```python
from build123d import *

# Parameters (mm, degrees)
F1_DEPTH = 15
F2_R     = 1
F3_R     = 1


with BuildPart() as f1:
    # F0 (on Front) → F1 (new body)
    with BuildSketch(Plane.XZ):
        Polygon((-4.5, 0), (-4.5, -18.7), (-2.75, -17.2), (-3.25, -7.2), (3.25, -7.2), (2.75, -17.2), (4.5, -18.7), (4.5, -1), (4.5, 0), align=None)
    extrude(amount=F1_DEPTH)

    # F2
    f2_edges = [f1.edges().sort_by_distance(p)[0] for p in [
        (-2.75, -7.5, -17.2),
        (-4.5, -7.5, 0),
        (4.5, -7.5, 0),
        (2.75, -7.5, -17.2),
    ]]
    fillet(f2_edges, radius=F2_R)

    # F3
    f3_edges = [f1.edges().sort_by_distance(p)[0] for p in [
        (-3.25, -7.5, -7.2),
        (3.25, -7.5, -7.2),
    ]]
    fillet(f3_edges, radius=F3_R)


solid = f1.part
```
Geometry check sheet. Reference: the model listing, model coordinates, mm. A direction names the side the tool comes from. Give positions to 0.01 mm unless a question says otherwise; leave off trailing zeros. Write each loop counter-clockwise with the first axis right and the second up, starting at its lowest first coordinate (ties: lowest second). Pieces come first, ordered by that corner, then holes. Notation, with made-up numbers: (56.5, 27) - (70.5, 27) arc R21 cw to (70.5, 57) - close; hole circle Ø5 at (-30, 12). An arc over 180 degrees is marked (long way). Use a Markdown table: item, result.
Q1. Thickness scan on L1, parallel to Z at x = 0, y = -11.5; L2, parallel to X at y = -10.5, z = -11; L3, parallel to X at y = -0.5, z = -16.25. Record the ranges inside material, lowest first. Write a range as [from, to].
Computed:
| item | result |
|---|---|
| L1 | z = [-7.2, 0] |
| L2 | x = [-4.5, -3.06], [3.06, 4.5] |
| L3 | x = [-4.5, -2.8], [2.8, 4.5] |
Q2. Go/stop test with flat-tipped pins: P1, Ø1, axis at x = 2.5, z = -6.5, coming from the +Y side; P2, Ø1, axis at x = -1, z = -9.5, coming from the -Y side. Record where each tip stops, or that it passes through.
Computed:
| item | result |
|---|---|
| P1 | stops at y = 0 |
| P2 | passes through |
Q3. Section check D-D, the plane z = -7.5. Enter the section's corners in (x, y), then the cut area to 3 significant figures.
Computed:
| item | result |
|---|---|
| outline | (-4.5, -15) - (-2.91, -15) - (-2.91, 0) - (-4.5, 0) - close; (2.91, -15) - (4.5, -15) - (4.5, 0) - (2.91, 0) - close |
| area | 47.6 mm² |
Q4. Section check C-C, the plane x = -1.25. Enter the section's corners in (y, z).
Computed:
| item | result |
|---|---|
| outline | (-15, -7.2) - (0, -7.2) - (0, 0) - (-15, 0) - close |
Q5. Draft check along Z on faces 1 (the face through (4.215, -7.605, -0.301)), 2 (the face through (-2.93, -7.6, -7.52)), 3 (the face through (-4.5, -7, -10)). Enter one of: pulls with the +Z half, pulls with the -Z half, needs draft (parallel to the pull), parting line crosses it, or undercut.
Computed:
| item | result |
|---|---|
| face 1 | pulls with the +Z half |
| face 2 | undercut |
| face 3 | needs draft |
Q6. Section check B-B, the plane y = -10.5. Enter the section's corners in (x, z), then the cut area to 3 significant figures.
Computed:
| item | result |
|---|---|
| outline | (-4.5, -18.7) - (-3.12, -17.52) arc R1 ccw to (-2.77, -16.71) - (-3.2, -8.25) arc R1 cw to (-2.2, -7.2) - (2.2, -7.2) arc R1 cw to (3.2, -8.25) - (2.77, -16.71) arc R1 ccw to (3.12, -17.52) - (4.5, -18.7) - (4.5, -1) arc R1 ccw to (3.5, 0) - (-3.5, 0) arc R1 ccw to (-4.5, -1) - close |
| area | 97.4 mm² |
Q7. Set-up check for faces 4 (the face through (-2.983, -7.395, -12.539)), 5 (the face through (0, 0, -7)), 6 (the face through (-3.8, -7.4, -18.1)): record each of +Z, -Z, +X, -X, +Y, -Y from which the full face is reachable in a straight line by a thin tool's end or side.
Computed:
| item | result |
|---|---|
| face 4 | +Y, -Y |
| face 5 | +Z, -Z, +X, -X, +Y |
| face 6 | -Z, +Y, -Y |
Q8. Section check A-A, the plane z = -15. Enter the section's corners in (x, y), then the cut area to 3 significant figures.
Computed:
| item | result |
|---|---|
| outline | (-4.5, -15) - (-2.86, -15) - (-2.86, 0) - (-4.5, 0) - close; (2.86, -15) - (4.5, -15) - (4.5, 0) - (2.86, 0) - close |
| area | 49.2 mm² |
